```python
from build123d import *

# Parameters (mm, degrees)
ESQUISSE1_R             = 10
BOSS_EXTRU_1_DEPTH      = 10
ESQUISSE2_R             = 2
BOSS_EXTRU_2_DEPTH      = 3
BOSS_EXTRU_2_DEPTH_BACK = 3
ESQUISSE4_R             = 1


with BuildPart() as part:
    # Esquisse1 → Boss.-Extru.1 (new body)
    with BuildSketch(Plane.XY):
        Circle(ESQUISSE1_R)
    extrude(amount=BOSS_EXTRU_1_DEPTH)

    # Balayage1: sweep along a path in Esquisse3
    with BuildLine(Plane(origin=(0, 0, 0), x_dir=(0, 0, -1), z_dir=(1, 0, 0))) as balayage1_path:
        Line((0, 0), (10, 0))
        ThreePointArc((10, 0), (11.414213562, -0.585786438), (12, -2))
        ThreePointArc((12, -2), (12.585786438, -3.414213562), (14, -4))
        Line((14, -4), (32, -4))
    # Esquisse2 → Balayage1 (sweep)
    with BuildSketch(Plane(origin=(0, 0, 0), x_dir=(-1, 0, 0), z_dir=(0, 0, -1))):
        Circle(ESQUISSE2_R)
    sweep(path=balayage1_path.line)

    # Esquisse4 → Boss.-Extru.2 (add, two sides: drawn at the far end of the back side and taken through both)
    with BuildSketch(Plane(origin=(0, 0, 0), x_dir=(0, 0, -1), z_dir=(1, 0, 0)).offset(-BOSS_EXTRU_2_DEPTH_BACK)):
        with Locations((18, -4)):
            Circle(ESQUISSE4_R)
        with Locations((30, -4)):
            Circle(ESQUISSE4_R)
    extrude(amount=BOSS_EXTRU_2_DEPTH + BOSS_EXTRU_2_DEPTH_BACK)


solid = part.part
```
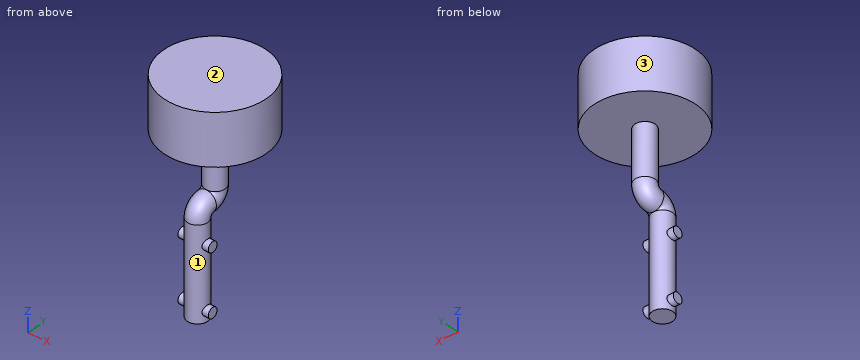
Input: part model. Units: mm. Frame: model coordinates. Face numbers are marked on the shaded views. Give positions to 0.01 mm unless a question says otherwise; leave off trailing zeros. Order: outer loops, then holes, each group sorted by start corner. A loop starts at its lowest first (then second) coordinate and runs counter-clockwise, first axis right, second up. Notation, with made-up numbers: M 3.25,41 L 14.25,41 A12 cw 14.25,50 Z; hole C 55.5,-22 d9. An arc over 180 degrees is marked long. Return JSON: item names as keys, results as strings.
1) Contact query for flat-ended pins moving along their axis: pin 1 (8 mm diameter, centred on y = -1, z = -2.5, fed in from +X); pin 2 (6 mm diameter, centred on y = -6.5, z = -12, fed in from -X); pin 3 (1 mm diameter, centred on y = -4, z = -30, fed in from -X); pin 4 (8 mm diameter, centred on x = 6, z = -1, fed in from +Y). Output: stop coordinate, or through.
Taken from the geometry:
{"pin 1": "stops at x = 10", "pin 2": "stops at x = -2", "pin 3": "stops at x = -3", "pin 4": "stops at y = 9.77"}
2) Section query A-A on z = -18. Output: boundary loops of the cut face in (x, y), and give its area (3 significant figures).
Taken from the geometry:
{"outline": "M -3,-5 L -1.73,-5 A2 ccw 1.73,-5 L 3,-5 L 3,-3 L 1.73,-3 A2 ccw -1.73,-3 L -3,-3 Z", "area": "16.9 mm2"}
3) Mould query, pull axis Z, two halves, no side actions, for the marked faces 1, 2 and 3. Classes: released by +Z, released by -Z, zero draft, split by the parting line, or undercut.
Taken from the geometry:
{"face 1": "undercut", "face 2": "released by +Z", "face 3": "zero draft"}
4) Line query: L1, parallel to Z at x = -7, y = -0.25; L2, parallel to Y at x = 7, z = 6; L3, parallel to Y at x = 9, z = 2.5. Output: solid intervals per line, ascending. Write a range as [from, to].
Taken from the geometry:
{"L1": "z = [0, 10]", "L2": "y = [-7.14, 7.14]", "L3": "y = [-4.36, 4.36]"}
5) Section query C-C on z = 1. Output: boundary loops of the cut face in (x, y), and give its area (3 significant figures).
Taken from the geometry:
{"outline": "C 0,0 d20", "area": "314 mm2"}
6) Section query D-D on y = 2.5. Output: boundary loops of the cut face in (x, z).
Taken from the geometry:
{"outline": "M -9.68,0 L 9.68,0 L 9.68,10 L -9.68,10 Z"}
7) Section query B-B on y = -8.5. Output: boundary loops of the cut face in (x, z), and give its area (3 significant figures).
Taken from the geometry:
{"outline": "M -5.27,0 L 5.27,0 L 5.27,10 L -5.27,10 Z", "area": "105 mm2"}
